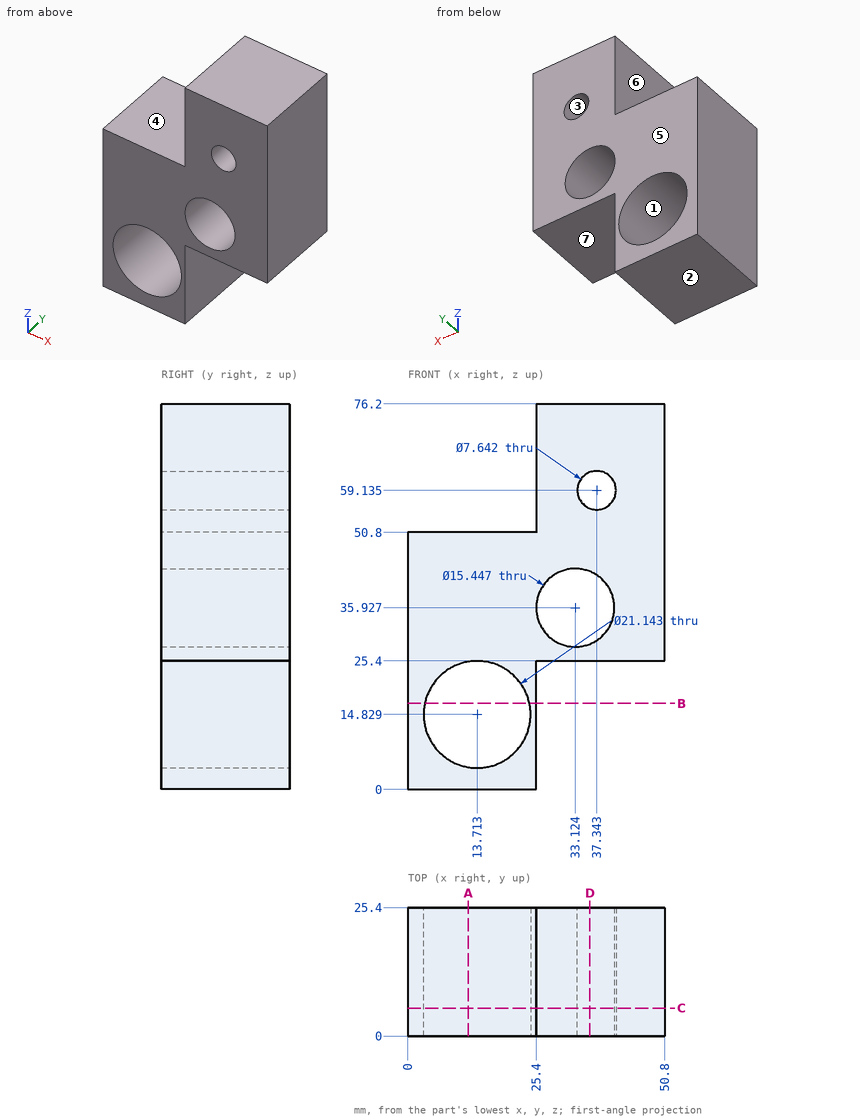
Drawing for the job (mm, zero at the part's lowest x, y, z). A direction names the side the tool comes from. Give positions to 0.01 mm unless a question says otherwise; leave off trailing zeros. Write each loop counter-clockwise with the first axis right and the second up, starting at its lowest first coordinate (ties: lowest second). Pieces come first, ordered by that corner, then holes. Notation, with made-up numbers: (58, 78.5) -> (82, 78.5) arc R22 ccw to (82, 91.5) -> close; hole circle Ø7 at (-30.75, -37.5). An arc over 180 degrees is marked (long way). Put each result on its own line as item: value. Start each with the question number.
Item 1: Cut at A-A (x = 12). List the corners of the cut face in (y, z).
Item 2: Cut at D-D (x = 36). List the corners of the cut face in (y, z) (1 decimal).
Item 3: Pin check, flat tips, straight feed: pin 1 Ø7.5 at (y, z) = (12, 67) entering from -X; pin 2 Ø7.5 at (y, z) = (17, 18.5) entering from +X; pin 3 Ø8 at (x, y) = (40, 17) entering from -Z; pin 4 Ø9.5 at (x, z) = (33.12, 35.93) entering from -Y. Stop position of each tip, or through.
Item 4: Cut at B-B (z = 17). List the corners of the cut face in (x, y).
Item 5: Which spindle directions (+Z, -Z, +X, -X, +Y, -Y) get a long thin tool onto all of the face, cutting with end or side? Do the marked faces 5, 6 and 7. Say none if no direction does.
Item 6: Cut at C-C (y = 5.5). List the corners of the cut face in (x, z) (1 decimal).
Item 7: Pull direction Z, two halves, no side cores. Call the marked faces 1, 2, 3 and 4: pulls with the +Z half, pulls with the -Z half, needs draft (parallel to the pull), parting line crosses it, or undercut.
Item 8: Wall check: L1, parallel to X at y = 1.5, z = 59 (1 decimal); L2, parallel to X at y = 18, z = 71; L3, parallel to Z at x = 44, y = 21.75. Give the ranges that are in metal, low to high. Write a range as [from, to].
Answer list:
1. outline: (0, 0) -> (25.4, 0) -> (25.4, 4.4) -> (0, 4.4) -> close; (0, 25.26) -> (25.4, 25.26) -> (25.4, 50.8) -> (0, 50.8) -> close
2. outline: (0, 25.4) -> (25.4, 25.4) -> (25.4, 28.8) -> (0, 28.8) -> close; (0, 43.1) -> (25.4, 43.1) -> (25.4, 55.6) -> (0, 55.6) -> close; (0, 62.7) -> (25.4, 62.7) -> (25.4, 76.2) -> (0, 76.2) -> close
3. pin 1: stops at x = 25.4
3. pin 2: stops at x = 25.4
3. pin 3: stops at z = 25.4
3. pin 4: passes through
4. outline: (0, 0) -> (3.37, 0) -> (3.37, 25.4) -> (0, 25.4) -> close; (24.06, 0) -> (25.4, 0) -> (25.4, 25.4) -> (24.06, 25.4) -> close
5. face 5: +Z, -Z, +X, -X, +Y
5. face 6: +Z, -X, +Y, -Y
5. face 7: -Z, +X, +Y, -Y
6. outline: (0, 0) -> (25.4, 0) -> (25.4, 25.4) -> (50.8, 25.4) -> (50.8, 76.2) -> (25.4, 76.2) -> (25.4, 50.8) -> (0, 50.8) -> close; hole circle Ø21.1 at (13.7, 14.8); hole circle Ø15.4 at (33.1, 35.9); hole circle Ø7.6 at (37.3, 59.1)
7. face 1: undercut
7. face 2: pulls with the -Z half
7. face 3: undercut
7. face 4: pulls with the +Z half
8. L1: x = [25.4, 33.5], [41.2, 50.8]
8. L2: x = [25.4, 50.8]
8. L3: z = [25.4, 76.2]
